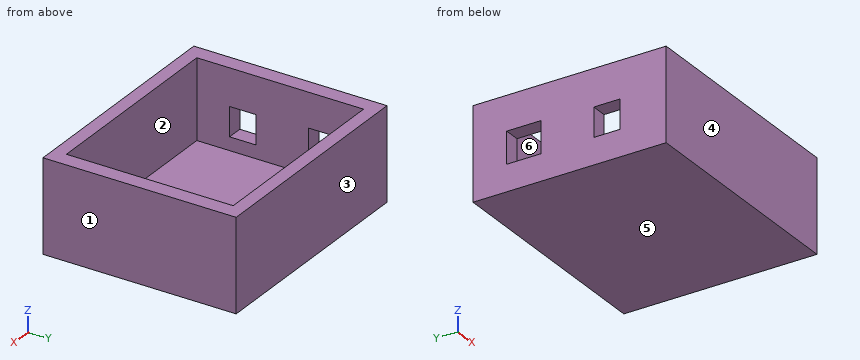
from build123d import *

# Parameters (mm, degrees)
F0_W      = 88.56
F0_H      = 73.2
F1_DEPTH  = 10
F1_FACE_W = 88.56
F1_FACE_H = 73.2
F2_DEPTH  = 25
F3_W      = 76.56
F3_H      = 63.2
F4_DEPTH  = 30
F6_W      = 13
F6_H      = 12
F6_W_2    = 10
F6_H_2    = 11
F7_DEPTH  = 25


with BuildPart() as f1:
    # F0 (on Top) → F1 (new body)
    with BuildSketch(Plane.XY):
        Rectangle(F0_W, F0_H)
    extrude(amount=-F1_DEPTH)

    # F1_face (on face) → F2 (join)
    with BuildSketch(Plane.XY):
        Rectangle(F1_FACE_W, F1_FACE_H)
    extrude(amount=F2_DEPTH)

    # F3 (on face) → F4 (cut)
    with BuildSketch(Plane.XY.offset(25)):
        Rectangle(F3_W, F3_H)
    extrude(amount=-F4_DEPTH, mode=Mode.SUBTRACT)

    # F6 (on face) → F7 (cut)
    with BuildSketch(Plane(origin=(-44.28, 0, 0), x_dir=(0, -1, 0), z_dir=(-1, 0, 0))):
        with Locations((-17.316721, 6)):
            Rectangle(F6_W, F6_H)
        with Locations((14.183279, 5.5)):
            Rectangle(F6_W_2, F6_H_2)
    extrude(amount=-F7_DEPTH, mode=Mode.SUBTRACT)


solid = f1.part
The model under review builds one solid part; all positions refer to its coordinate system, in mm. Face numbers are marked on the shaded views. A direction names the side the tool comes from. Give positions to 0.01 mm unless a question says otherwise; leave off trailing zeros. Loops run counter-clockwise (first coordinate to the right, second up) from the corner with the lowest first, then second, coordinate; pieces in that order, holes last. Notation, with made-up numbers: (-18.5, 54) -> (21.5, 54) arc R19 ccw to (21.5, 75) -> close; hole circle Ø5 at (66, -6.75). An arc over 180 degrees is marked (long way). Put each result on its own line as item: value. Start each with the question number.
1. Mouldability with a two-part tool opening along Y and no side actions: class the marked faces 3, 4, 5 and 6 as released by +Y, released by -Y, zero draft, split by the parting line, or undercut.
2. We need section C-C on y = 25.5. State the section outline as (x, z) points.
3. For the marked faces 1 and 2, list the 3-axis set-ups (+Z, -Z, +X, -X, +Y, -Y) from which the entire face can be reached by the end or side of a thin tool; tool diameter is ignored.
4. Wall thickness on probe 1 along X at (y, z) = (-23.5, 12.5); probe 2 along Y at (x, z) = (24.5, -1.5); probe 3 along Z at (x, y) = (-17, 1): over which ranges is each line inside the solid? List them lowest first.
5. Clearance check with a flat-ended pin moving along its axis: P1, Ø5, axis at x = 4.5, y = 2, coming from the +Z side. State where the tip first meets the part, or that it passes through.
6. We need section A-A on z = 6. State the section outline as (x, y) points, then the cut area to 3 significant figures.
7. We need section D-D on x = 20. State the section outline as (y, z) points, then the cut area to 3 significant figures.
8. We need section B-B on z = -2.5. State the section outline as (x, y) points.
Determined:
1. face 3: released by +Y
1. face 4: released by -Y
1. face 5: zero draft
1. face 6: undercut
2. outline: (-44.28, -10) -> (44.28, -10) -> (44.28, 25) -> (38.28, 25) -> (38.28, -5) -> (-38.28, -5) -> (-38.28, 25) -> (-44.28, 25) -> close
3. face 1: +Z, -Z, +X, +Y, -Y
3. face 2: +Z
4. probe 1: -44.28 to -38.28, 38.28 to 44.28
4. probe 2: -36.6 to -31.6, 31.6 to 36.6
4. probe 3: -10 to -5
5. P1: z = -5
6. outline: (-44.28, -36.6) -> (44.28, -36.6) -> (44.28, 36.6) -> (-44.28, 36.6) -> (-44.28, 23.82) -> (-38.28, 23.82) -> (-38.28, 31.6) -> (38.28, 31.6) -> (38.28, -31.6) -> (-38.28, -31.6) -> (-38.28, -19.18) -> (-44.28, -19.18) -> close; (-44.28, -9.18) -> (-38.28, -9.18) -> (-38.28, 10.82) -> (-44.28, 10.82) -> close
6. area: 1,510 mm^2
7. outline: (-36.6, -10) -> (36.6, -10) -> (36.6, 25) -> (31.6, 25) -> (31.6, -5) -> (-31.6, -5) -> (-31.6, 25) -> (-36.6, 25) -> close
7. area: 666 mm^2
8. outline: (-44.28, -36.6) -> (44.28, -36.6) -> (44.28, 36.6) -> (-44.28, 36.6) -> close; hole (-38.28, -31.6) -> (38.28, -31.6) -> (38.28, 31.6) -> (-38.28, 31.6) -> close
